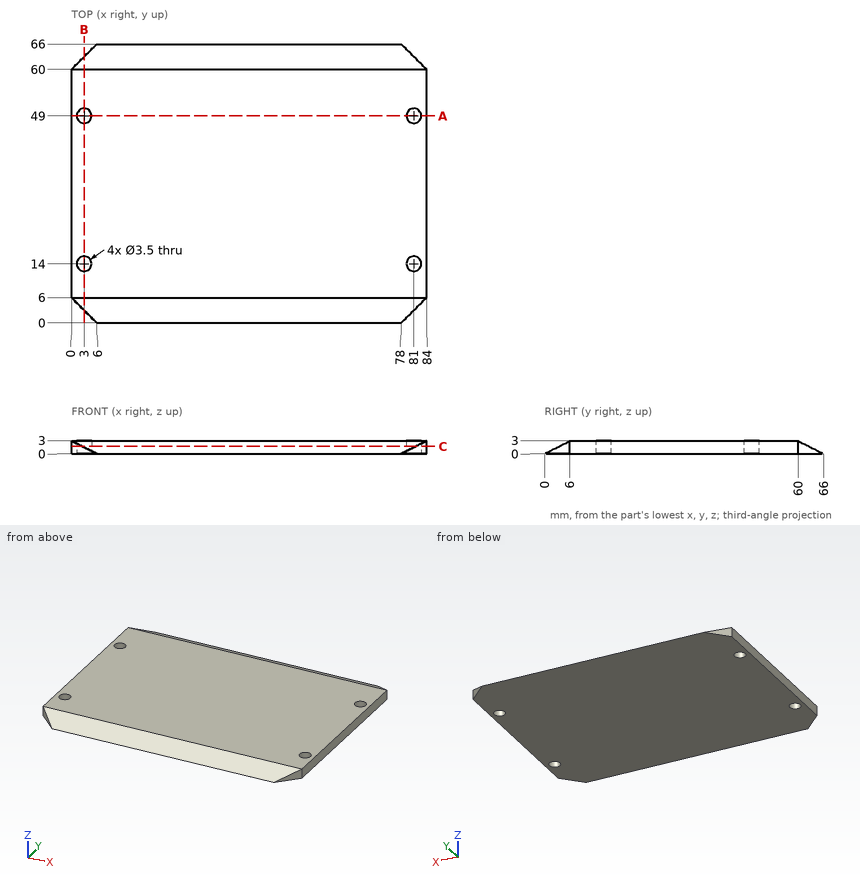
Job drawing, mm, ordinate dimensions from the low corner. One solid piece. Give positions to 0.01 mm unless a question says otherwise; leave off trailing zeros. Write each loop counter-clockwise with the first axis right and the second up, starting at its lowest first coordinate (ties: lowest second). Pieces come first, ordered by that corner, then holes. Notation, with made-up numbers: M -9.75,-31 L 32.25,-31 A20 ccw 32.25,-13 Z; hole C -21,40 d1. An arc over 180 degrees is marked long. Put each result on its own line as item: value. Start each with the question number.
(1) Flat gauge pin, fed straight in: pin 1 Ø2 at (x, y) = (3, 49) entering from +Z. Where does the tip first touch, or does it go through?
(2) Band-saw the part on A-A, the plane y = 49. Write the cut outline in (x, z), and give its area (3 significant figures).
(3) Band-saw the part on C-C, the plane z = 1.7. Write the cut outline in (x, y), and give its area (3 significant figures).
(4) Probe L1, parallel to Y at x = 81, z = 1.4; L2, parallel to X at y = 50, z = 2.2; L3, parallel to Y at x = 3, z = 2.05. List the from-to ranges inside material, lowest first.
(5) Band-saw the part on B-B, the plane x = 3. Write the cut outline in (y, z), and give its area (4 significant figures).
Response values:
1. pin 1: passes through
2. outline: M 0,0 L 1.25,0 L 1.25,3 L 0,3 Z; M 4.75,0 L 79.25,0 L 79.25,3 L 4.75,3 Z; M 82.75,0 L 84,0 L 84,3 L 82.75,3 Z
2. area: 231 mm2
3. outline: M 0,6 L 2.6,3.4 L 81.4,3.4 L 84,6 L 84,60 L 81.4,62.6 L 2.6,62.6 L 0,60 Z; hole C 3,14 d3.5; hole C 3,49 d3.5; hole C 81,14 d3.5; hole C 81,49 d3.5
3. area: 4,920 mm2
4. L1: y = 3 to 12.25, 15.75 to 47.25, 50.75 to 63
4. L2: x = 0 to 1.56, 4.44 to 79.56, 82.44 to 84
4. L3: y = 4.1 to 12.25, 15.75 to 47.25, 50.75 to 61.9
5. outline: M 3,0 L 12.25,0 L 12.25,3 L 6,3 L 3,1.5 Z; M 15.75,0 L 47.25,0 L 47.25,3 L 15.75,3 Z; M 50.75,0 L 63,0 L 63,1.5 L 60,3 L 50.75,3 Z
5. area: 154.5 mm2
